Design review of the part built by this model. Coordinates are the model's own, in mm. A direction names the side the tool comes from. Coordinates: 2 decimals unless noted, no trailing zeros. Write each loop counter-clockwise with the first axis right and the second up, starting at its lowest first coordinate (ties: lowest second). Pieces come first, ordered by that corner, then holes. Notation, with made-up numbers: (4, 68.25) -> (51, 68.25) arc R14 cw to (51, 95.25) -> close; hole circle Ø2 at (10.5, 19). An arc over 180 degrees is marked (long way). Answer in a Markdown table with one row per item. Add a question column.
Item 1: Draft analysis for pull direction X (two halves, no side actions). For faces 1 (the face through (0.19, -21.32, 3.45)), 2 (the face through (0, 40, 3)), 3 (the face through (14.781, -25.855, 3.451)), 4 (the face through (-18.559, 10.496, 3.451)), state which applies: released by +X, released by -X, zero draft, split by the parting line, or undercut.
Item 2: Take a section at D-D, the plane y = 30.5. Write out the cut boundary in (x, z).
Item 3: For faces 5 (the face through (-15, 26, 3)), 6 (the face through (15, 26, 3)), 7 (the face through (25.975, -28.126, 3.549)), list the 3-axis set-ups (+Z, -Z, +X, -X, +Y, -Y) from which the entire face can be reached by the end or side of a thin tool; tool diameter is ignored.
Item 4: Take a section at C-C, the plane y = -12. Write out the cut boundary in (x, z), and give its area (3 significant figures).
Item 5: Take a section at B-B, the plane z = 3. Write out the cut boundary in (x, y).
Item 6: Clearance check with flat-ended pins moving along their axes: P1, Ø2, axis at y = 26.5, z = 4.5, coming from the -X side; P2, Ø4, axis at y = 0, z = 2.5, coming from the +X side; P3, Ø2, axis at y = 25, z = 2.5, coming from the +X side. State where each tip first meets the part, or that it passes through.
Item 7: To check wall thickness, follow line 1 (Y direction, x = 8, z = 4.5); line 2 (Y direction, x = -4.5, z = 4.75); line 3 (X direction, y = -6, z = 4.75). State the ranges of each line that lie inside material, in increasing order.
Item 8: Take a section at A-A, the plane x = 21. Write out the cut boundary in (y, z).
from build123d import *

# Parameters (mm, degrees)
F1_DEPTH = 7
F3_ANGLE = 120
F4_ANGLE = 240
F6_R     = 25.8564064606
F7_R     = 25.856
F8_R     = 25.856
F9_R     = 12.0710678119
F10_R    = 12.071
F11_R    = 12.071
F12_R    = 12.071
F13_R    = 12.071
F14_R    = 12.071


with BuildPart() as f1:
    # F0 (on Top) → F1 (new body)
    with BuildSketch(Plane.XY):
        with BuildLine():
            ThreePointArc((-11, 0), (-7.7781745931, 7.7781745931), (0, 11))
            Line((0, 11), (0, 14.1644365489))
            ThreePointArc((0, 14.1644365489), (-11, 25.1644365489), (0, 36.1644365489))
            Line((0, 36.1644365489), (0, 40))
            Line((0, 40), (-15, 40))
            Line((-15, 40), (-15, 0))
            Line((-15, 0), (-11, 0))
        make_face()
        with BuildLine():
            ThreePointArc((0, 11), (7.7781745931, 7.7781745931), (11, 0))
            Line((11, 0), (15, 0))
            Line((15, 0), (15, 40))
            Line((15, 40), (0, 40))
            Line((0, 40), (0, 36.1644365489))
            ThreePointArc((0, 36.1644365489), (7.7781745931, 32.942611142), (11, 25.1644365489))
            ThreePointArc((11, 25.1644365489), (7.7781745931, 17.3862619559), (0, 14.1644365489))
            Line((0, 14.1644365489), (0, 11))
        make_face()
    extrude(amount=F1_DEPTH)


with BuildPart() as f3_1:
    # F3: copy of F1
    add(f1.part.rotate(Axis((0, 0, 22.2638938576), (0, 0, 1)), F3_ANGLE))


with BuildPart() as f4_1:
    # F4: copy of F1
    add(f1.part.rotate(Axis((0, 0, 22.2638938576), (0, 0, 1)), F4_ANGLE))


with BuildPart() as f1_1:
    add(f1.part)

    # F5: union F3_1, F4_1
    add(f3_1.part)
    add(f4_1.part)

    # F6
    f6_edges = [f1_1.edges().sort_by_distance(p)[0] for p in [
        (0, -17.320508, 3.5),
    ]]
    fillet(f6_edges, radius=F6_R)

    # F7
    f7_edges = [f1_1.edges().sort_by_distance(p)[0] for p in [
        (-15, 8.660254, 3.5),
    ]]
    fillet(f7_edges, radius=F7_R)

    # F8
    f8_edges = [f1_1.edges().sort_by_distance(p)[0] for p in [
        (15, 8.660254, 3.5),
    ]]
    fillet(f8_edges, radius=F8_R)

    # F9
    f9_edges = [f1_1.edges().sort_by_distance(p)[0] for p in [
        (-27.141016, -32.990381, 3.5),
    ]]
    fillet(f9_edges, radius=F9_R)

    # F10
    f10_edges = [f1_1.edges().sort_by_distance(p)[0] for p in [
        (-42.141016, -7.009619, 3.5),
    ]]
    fillet(f10_edges, radius=F10_R)

    # F11
    f11_edges = [f1_1.edges().sort_by_distance(p)[0] for p in [
        (-15, 40, 3.5),
    ]]
    fillet(f11_edges, radius=F11_R)

    # F12
    f12_edges = [f1_1.edges().sort_by_distance(p)[0] for p in [
        (15, 40, 3.5),
    ]]
    fillet(f12_edges, radius=F12_R)

    # F13
    f13_edges = [f1_1.edges().sort_by_distance(p)[0] for p in [
        (27.141016, -32.990381, 3.5),
    ]]
    fillet(f13_edges, radius=F13_R)

    # F14
    f14_edges = [f1_1.edges().sort_by_distance(p)[0] for p in [
        (42.141016, -7.009619, 3.5),
    ]]
    fillet(f14_edges, radius=F14_R)


solid = f1_1.part
Answers:
| question | item | result |
|---|---|---|
| 1 | face 1 | undercut |
| 1 | face 2 | zero draft |
| 1 | face 3 | undercut |
| 1 | face 4 | released by -X |
| 2 | outline | (-14.72, 0) -> (-9.62, 0) -> (-9.62, 7) -> (-14.72, 7) -> close; (9.62, 0) -> (14.72, 0) -> (14.72, 7) -> (9.62, 7) -> close |
| 3 | face 5 | +Z, -Z, -X, +Y |
| 3 | face 6 | +Z, -Z, +X, +Y |
| 3 | face 7 | +Z, -Z, -Y |
| 4 | outline | (-37.71, 0) -> (-32.78, 0) -> (-32.78, 7) -> (-37.71, 7) -> close; (-10.81, 0) -> (10.81, 0) -> (10.81, 7) -> (-10.81, 7) -> close; (32.78, 0) -> (37.71, 0) -> (37.71, 7) -> (32.78, 7) -> close |
| 4 | area | 220 mm^2 |
| 5 | outline | (-36.11, -17.46) -> (-33.18, -22.54) arc R12.07 ccw to (-16.69, -26.95) -> (-12.93, -24.78) arc R25.86 cw to (12.93, -24.78) -> (16.69, -26.95) arc R12.07 ccw to (33.18, -22.54) -> (36.11, -17.46) arc R12.07 ccw to (31.69, -0.97) -> (27.93, 1.2) arc R25.86 cw to (15, 23.59) -> (15, 27.93) arc R12.07 ccw to (2.93, 40) -> (-2.93, 40) arc R12.07 ccw to (-15, 27.93) -> (-15, 23.59) arc R25.86 cw to (-27.93, 1.2) -> (-31.69, -0.97) arc R12.07 ccw to start; hole circle Ø22 at (-21.79, -12.58); hole circle Ø22 at (0, 0); hole circle Ø22 at (0, 25.16); hole circle Ø22 at (21.79, -12.58) |
| 6 | P1 | stops at x = -15 |
| 6 | P2 | stops at x = 33.19 |
| 6 | P3 | stops at x = 15 |
| 7 | line 1 | y = -22.59 to -7.55, 7.55 to 17.61, 32.71 to 38.88 |
| 7 | line 2 | y = -21.72 to -10.04, 10.04 to 15.13, 35.2 to 39.9 |
| 7 | line 3 | x = -36.43 to -30.61, -12.98 to -9.22, 9.22 to 12.98, 30.61 to 36.43 |
| 8 | outline | (-28.45, 0) -> (-23.55, 0) -> (-23.55, 7) -> (-28.45, 7) -> close; (-1.61, 0) -> (7.03, 0) -> (7.03, 7) -> (-1.61, 7) -> close |
